Model file for the job. Use its own axes, mm. A direction names the side the tool comes from. Coordinates: 2 decimals unless noted, no trailing zeros. Order: outer loops, then holes, each group sorted by start corner. A loop starts at its lowest first (then second) coordinate and runs counter-clockwise, first axis right, second up.
from build123d import *

# Parameters (mm, degrees)
F0_W     = 365
F0_H     = 185
F1_DEPTH = 1600
F2_W     = 75
F2_H     = 75
F3_DEPTH = 380
F4_W     = 115
F4_H     = 185
F5_DEPTH = 325
F7_DEPTH = 185.001


with BuildPart() as f1:
    # F0 (on Top) → F1 (new body)
    with BuildSketch(Plane.XY):
        Rectangle(F0_W, F0_H)
    extrude(amount=F1_DEPTH)

    # F2 (on Front) → F3 (join)
    with BuildSketch(Plane.XZ):
        with Locations((-145, 1025)):
            Rectangle(F2_W, F2_H)
        with Locations((145, 1025)):
            Rectangle(F2_W, F2_H)
    extrude(amount=F3_DEPTH)

    # F4 (on face) → F5 (cut)
    with BuildSketch(Plane.XY.offset(1600)):
        with Locations((-125, 0)):
            Rectangle(F4_W, F4_H)
        with Locations((125, 0)):
            Rectangle(F4_W, F4_H)
    extrude(amount=-F5_DEPTH, mode=Mode.SUBTRACT)

    # F6 (on face) → F7 (cut, through all)
    with BuildSketch(Plane.XZ.offset(92.5)):
        Polygon((-102.5, 0), (-182.5, 700), (-182.5, 0), align=None)
        Polygon((182.5, 0), (182.5, 700), (102.5, 0), align=None)
    extrude(amount=-F7_DEPTH, mode=Mode.SUBTRACT)


solid = f1.part
Q1. Cut at B-B, the plane x = 123.5. List the corners of the cut face in (y, z).
Established:
outline: (-380, 987.5) - (-92.5, 987.5) - (-92.5, 183.75) - (92.5, 183.75) - (92.5, 1275) - (-92.5, 1275) - (-92.5, 1062.5) - (-380, 1062.5) - close
Q2. Cut at D-D, the plane y = 53. List the corners of the cut face in (x, z).
Established:
outline: (-182.5, 700) - (-102.5, 0) - (102.5, 0) - (182.5, 700) - (182.5, 1275) - (67.5, 1275) - (67.5, 1600) - (-67.5, 1600) - (-67.5, 1275) - (-182.5, 1275) - close
Q3. Cut at C-C, the plane z = 724. List the corners of the cut face in (x, y).
Established:
outline: (-182.5, -92.5) - (182.5, -92.5) - (182.5, 92.5) - (-182.5, 92.5) - close
Q4. Drop flat-ended pins along their axis: P1, Ø1.5, axis at x = 136, y = -116.5, coming from the +Z side; P2, Ø1, axis at x = 76, z = 390, coming from the -Y side; P3, Ø8, axis at x = 64.5, y = 41.5, coming from the -Z side; P4, Ø4, axis at y = 36, z = 370.5, coming from the +X side. Give the stop position or say it passes through.
Established:
P1: stops at z = 1062.5
P2: stops at y = -92.5
P3: stops at z = 0
P4: stops at x = 145.07
Q5. Which spindle directions (+Z, -Z, +X, -X, +Y, -Y) get a long thin tool onto all of the face, cutting with end or side? Do faces 1 (the face through (67.5, -1, 1440)), 2 (the face through (-126, 1, 1275)), 3 (the face through (107.5, -234, 1024)), 4 (the face through (-146, -234, 987.5)). Say none if no direction does.
Established:
face 1: +Z, +X, +Y, -Y
face 2: +Z, -X, +Y, -Y
face 3: +Z, -Z, -Y
face 4: -Z, +X, -X, -Y
Q6. Mould opens along X. For faces 5 (the face through (-67.5, -1, 1440)), 6 (the face through (-107.5, -234, 1024)), 7 (the face through (-1, 1, 1600)) say: pulls with the +X half, pulls with the -X half, needs draft (parallel to the pull), parting line crosses it, or undercut.
Established:
face 5: pulls with the -X half
face 6: undercut
face 7: needs draft
Q7. Probe line 1 (Y direction, x = -23, z = 932); line 2 (Z direction, x = -98.5, y = -4); line 3 (X direction, y = 41.5, z = 602). List the from-to ranges inside material, lowest first.
Established:
line 1: y = -92.5 to 92.5
line 2: z = 0 to 1275
line 3: x = -171.3 to 171.3
Q8. Cut at A-A, the plane y = -300. List the corners of the cut face in (x, z).
Established:
outline: (-182.5, 987.5) - (-107.5, 987.5) - (-107.5, 1062.5) - (-182.5, 1062.5) - close; (107.5, 987.5) - (182.5, 987.5) - (182.5, 1062.5) - (107.5, 1062.5) - close
